from build123d import *

# Parameters (mm, degrees)
F1_DEPTH = 12
F2_R     = 1.6
F3_DEPTH = 2
F4_DEPTH = 10.051
F5_R     = 1.6
F6_DEPTH = 25
F7_SIZE  = 2


with BuildPart() as f1:
    # F0 (on Top) → F1 (new body)
    with BuildSketch(Plane.XY):
        with BuildLine():
            ThreePointArc((2.9563490998, -0.75), (-3.05, 0), (2.9563490998, 0.75))
            Line((2.9563490998, 0.75), (10.9563490998, 0.75))
            Line((10.9563490998, 0.75), (10.9563490998, 3.75))
            Line((10.9563490998, 3.75), (4.0914545091, 3.75))
            ThreePointArc((4.0914545091, 3.75), (-5.5212512675, 0.5641670326), (3.2484611742, -4.5))
            Line((3.2484611742, -4.5), (16.9563490998, -4.5))
            Line((16.9563490998, -4.5), (16.9563490998, -0.75))
            Line((16.9563490998, -0.75), (2.9563490998, -0.75))
        make_face()
    extrude(amount=F1_DEPTH)

    # F2 (on face) → F3 (cut)
    with BuildSketch(Plane.XZ.offset(4.5)):
        Polygon((9.8514510462, 7.6111043179), (7.0296988427, 9.2763138649), (4.1767089707, 7.665209547), (4.1454713021, 4.3888956821), (6.9672235056, 2.7236861351), (9.8202133776, 4.334790453), align=None)
        with Locations((6.9984611742, 6)):
            Circle(F2_R, mode=Mode.SUBTRACT)
        with Locations((6.9984611742, 6)):
            Circle(F2_R)
    extrude(amount=-F3_DEPTH, mode=Mode.SUBTRACT)

    # F2 (on face) → F4 (cut, through all)
    with BuildSketch(Plane.XZ.offset(4.5)):
        with Locations((6.9984611742, 6)):
            Circle(F2_R)
    extrude(amount=-F4_DEPTH, mode=Mode.SUBTRACT)

    # F5 (on face) → F6 (cut)
    with BuildSketch(Plane(origin=(0, 3.75, 0), x_dir=(-1, 0, 0), z_dir=(0, 1, 0))):
        with Locations((-6.9984611742, 6)):
            Circle(F5_R)
        with BuildLine():
            ThreePointArc((-4.0914545091, 4.5467924273), (-3.8353715721, 5.2534317384), (-3.7484611742, 6))
            ThreePointArc((-3.7484611742, 6), (-3.8353715721, 6.7465682616), (-4.0914545091, 7.4532075727))
            Line((-4.0914545091, 7.4532075727), (-4.0914545091, 4.5467924273))
        make_face()
    extrude(amount=F6_DEPTH, mode=Mode.SUBTRACT)

    # F7
    f7_edges = [f1.edges().sort_by_distance(p)[0] for p in [
        (16.956349, -2.625, 12),
        (16.956349, -2.625, 0),
        (10.956349, 2.25, 0),
        (10.956349, 2.25, 12),
    ]]
    chamfer(f7_edges, length=F7_SIZE)


solid = f1.part
Model file for the job. Use its own axes, mm. A direction names the side the tool comes from. Give positions to 0.01 mm unless a question says otherwise; leave off trailing zeros. Loops run counter-clockwise (first coordinate to the right, second up) from the corner with the lowest first, then second, coordinate; pieces in that order, holes last.
Item 1: Slice it at C-C (z = 9.5). Write the cut outline in (x, y), plus the area to 3 significant figures.
Check values:
outline: (2.96, -0.75) arc R3.05 cw (long way) to (2.96, 0.75) - (10.96, 0.75) - (10.96, 3.75) - (4.09, 3.75) arc R5.55 ccw (long way) to (3.25, -4.5) - (16.96, -4.5) - (16.96, -0.75) - close
area: 128 mm2
Item 2: Which spindle directions (+Z, -Z, +X, -X, +Y, -Y) get a long thin tool onto all of the face, cutting with end or side? Do faces 1 (the face through (5.62, -3.51, 8.48)), 2 (the face through (9.97, 2.229, 10.986)), 3 (the face through (9.942, 2.229, 0.986)). Say none if no direction does.
Check values:
face 1: -Y
face 2: +Z, +X, +Y
face 3: -Z, +X, +Y
Item 3: Drop flat-ended pins along their axis: P1, Ø1, axis at x = -1.5, y = -1, coming from the -Z side; P2, Ø6.5, axis at x = 9, z = 6, coming from the -Y side; P3, Ø4, axis at x = 7, z = 6, coming from the +Y side; P4, Ø0.9, axis at y = 2.5, z = 5.5, coming from the +X side. Give the stop position or say it passes through.
Check values:
P1: passes through
P2: stops at y = -4.5
P3: stops at y = 3.75
P4: stops at x = 10.96
Item 4: Mould opens along X. For faces 4 (the face through (5.537, -3.514, 3.568)), 5 (the face through (5, 0.75, 6)), 6 (the face through (-5.5, 0.74, 5.92)), 7 (the face through (15.97, -2.651, 10.986)) say: +X half, -X half, draft (parallel to the pull), parting line (faces both ways), or undercut.
Check values:
face 4: undercut
face 5: draft
face 6: parting line
face 7: +X half
Item 5: Slice it at A-A (x = 0). Write the cut outline in (y, z).
Check values:
outline: (-5.55, 0) - (-3.05, 0) - (-3.05, 12) - (-5.55, 12) - close; (3.05, 0) - (5.55, 0) - (5.55, 12) - (3.05, 12) - close
Item 6: Drill centre lines: line 1 along X through (y, z) = (1.75, 6.5); line 2 along Y through (x, z) = (7.5, 2.5); line 3 along X through (y, z) = (2.4, 6). Where is each one in solid material? Low to high.
Check values:
line 1: x = -5.27 to -2.5, 2.5 to 5.48, 8.52 to 10.96
line 2: y = -4.5 to -0.75, 0.75 to 3.75
line 3: x = -5 to -1.88, 1.88 to 5.4, 8.6 to 10.96
Item 7: Slice it at B-B (y = 1.5). Write the cut outline in (x, z).
Check values:
outline: (-5.34, 0) - (-2.66, 0) - (-2.66, 12) - (-5.34, 12) - close; (2.66, 0) - (8.96, 0) - (10.96, 2) - (10.96, 10) - (8.96, 12) - (2.66, 12) - close; hole circle Ø3.2 at (7, 6)
Item 8: Slice it at D-D (x = 7.5). Write the cut outline in (y, z), plus the area to 3 significant figures.
Check values:
outline: (-4.5, 0) - (-0.75, 0) - (-0.75, 4.48) - (-2.5, 4.48) - (-2.5, 3.02) - (-4.5, 3.02) - close; (-4.5, 9) - (-2.5, 9) - (-2.5, 7.52) - (-0.75, 7.52) - (-0.75, 12) - (-4.5, 12) - close; (0.75, 0) - (3.75, 0) - (3.75, 4.48) - (0.75, 4.48) - close; (0.75, 7.52) - (3.75, 7.52) - (3.75, 12) - (0.75, 12) - close
area: 54.6 mm2
